from build123d import *

# Parameters (mm, degrees)
BOSS_EXTRUDE1_DEPTH = 20
SKETCH3_R           = 0.8
CUT_EXTRUDE1_DEPTH  = 6
SKETCH2_R           = 1
BOSS_EXTRUDE2_DEPTH = 5
LPATTERN1_COUNT     = 15
LPATTERN1_PITCH     = 0.4
LPATTERN2_COUNT     = 13
LPATTERN2_PITCH     = 0.4


with BuildPart() as part:
    # Sketch1 → Boss-Extrude1 (new body)
    with BuildSketch(Plane(origin=(0, 0, 0), x_dir=(1, 0, 0), z_dir=(0, 1, 0))):
        Polygon((2.309401077, 0), (1.154700538, 2), (-1.154700538, 2), (-2.309401077, 0), (-1.154700538, -2), (1.154700538, -2), align=None)
    extrude(amount=BOSS_EXTRUDE1_DEPTH)

    # Sketch3 → Cut-Extrude1 (cut)
    with BuildSketch(Plane.XZ):
        Circle(SKETCH3_R)
    extrude(amount=-CUT_EXTRUDE1_DEPTH, mode=Mode.SUBTRACT)

    # Sketch2 → Boss-Extrude2 (add)
    with BuildSketch(Plane(origin=(0, 20, 0), x_dir=(1, 0, 0), z_dir=(0, 1, 0))):
        Circle(SKETCH2_R)
    extrude(amount=BOSS_EXTRUDE2_DEPTH)

    # Sketch5 → Cut-Revolve1 (revolve, cut)
    with BuildSketch(Plane.XY):
        Polygon((0.38, 0.2), (0.38, -0.2), (0.78, -0.2), (1.126410162, 0), (0.78, 0.2), align=None)
    cut_revolve1 = revolve(axis=Axis((0, 0, 0), (0, 1, 0)), mode=Mode.SUBTRACT)

    # LPattern1: Cut-Revolve1 ×15
    with Locations(*[(0, i * LPATTERN1_PITCH, 0) for i in range(1, LPATTERN1_COUNT)]):
        add(cut_revolve1, mode=Mode.SUBTRACT)

    # Sketch6 → Cut-Revolve2 (revolve, cut)
    with BuildSketch(Plane.XY):
        Polygon((1.446410162, 25.2), (1.446410162, 24.8), (1.046410162, 24.8), (0.7, 25), (1.046410162, 25.2), align=None)
    cut_revolve2 = revolve(axis=Axis((0, 0, 0), (0, 1, 0)), mode=Mode.SUBTRACT)

    # LPattern2: Cut-Revolve2 ×13
    with Locations(*[(0, -i * LPATTERN2_PITCH, 0) for i in range(1, LPATTERN2_COUNT)]):
        add(cut_revolve2, mode=Mode.SUBTRACT)


solid = part.part
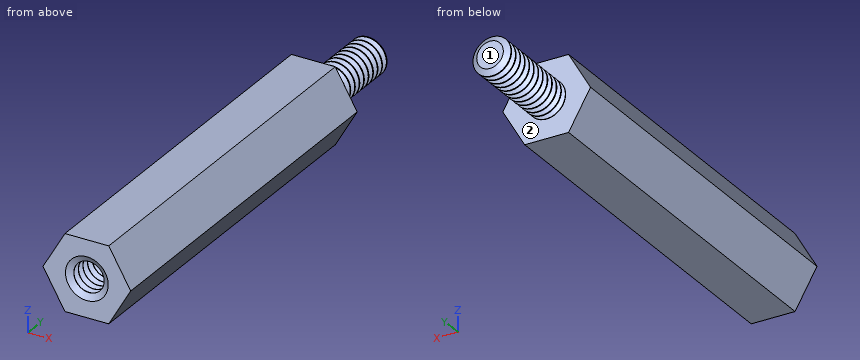
Here's how the part is built. I have some questions about the finished solid (model axes, mm). Face numbers are marked on the shaded views. A direction names the side the tool comes from. Round coordinates to 2 decimals unless told otherwise and drop trailing zeros. Loops run counter-clockwise (first coordinate to the right, second up) from the corner with the lowest first, then second, coordinate; pieces in that order, holes last.
1. If I drill on line 1 along Z through (x, y) = (0, 5.95); line 2 along Y through (x, z) = (1.35, -0.8); line 3 along Y through (x, z) = (-0.35, -0.25), over which ranges is the centre line in solid material (lowest first)?
Answer list:
line 1: z = -2 to -0.8, 0.8 to 2
line 2: y = 0 to 20
line 3: y = 6 to 25
2. For P1, Ø1.8, axis at x = 0, z = 0, coming from the -Y side; P2, Ø1.4, axis at x = 0, z = 0, coming from the -Y side; P3, Ø1, axis at y = 21.5, z = 0, coming from the +X side, each with a flat end and sliding along its axis, tell me the tip position at first contact or that it passes through.
Answer list:
P1: stops at y = 0.13
P2: stops at y = 6
P3: stops at x = 1
3. If we section it at B-B on z = 1.55: Write out the boundary of the cut face in (x, y).
Answer list:
outline: (-1.41, 0) - (1.41, 0) - (1.41, 20) - (-1.41, 20) - close
4. Which directions (+Z, -Z, +X, -X, +Y, -Y) give clear straight access to the entire face, cutting with the end or side of a thin tool? Please do the marked faces 1 and 2.
Answer list:
face 1: +Z, -Z, +X, -X, +Y
face 2: +Y
5. If we section it at A-A on y = 14: Write out the boundary of the cut face in (x, z), plus the area to 3 significant figures.
Answer list:
outline: (-2.31, 0) - (-1.15, -2) - (1.15, -2) - (2.31, 0) - (1.15, 2) - (-1.15, 2) - close
area: 13.9 mm2
